```python
from build123d import *

# Parameters (mm, degrees)
SKETCH_1_R               = 2
EXTRUDE_1_DEPTH          = 15
SKETCH_2_R               = 2.5
EXTRUDE_2_DEPTH          = 4
SKETCH_3_R               = 3
EXTRUDE_3_DEPTH          = 3
SKETCH_4_R               = 9
EXTRUDE_4_DEPTH          = 3
SKETCH_5_R               = 3
EXTRUDE_5_DEPTH          = 20
SKETCH_8_R               = 2
EXTRUDE_6_DEPTH          = 4
HOLE_WIZARD_M3_2_D       = 2.5
PATTERN_CIRCULAR_2_COUNT = 4
CHAMFER_1_SIZE           = 0.3


with BuildPart() as part:
    # 草图1 → 凸台-拉伸1 (new body)
    with BuildSketch(Plane(origin=(0, 0, 0), x_dir=(0, 0, -1), z_dir=(1, 0, 0))):
        Circle(SKETCH_1_R)
    extrude(amount=EXTRUDE_1_DEPTH)

    # 草图2 → 凸台-拉伸2 (add)
    with BuildSketch(Plane(origin=(15, 0, 0), x_dir=(0, 0, -1), z_dir=(1, 0, 0))):
        Circle(SKETCH_2_R)
    extrude(amount=EXTRUDE_2_DEPTH)

    # 草图3 → 凸台-拉伸3 (add)
    with BuildSketch(Plane(origin=(19, 0, 0), x_dir=(0, 0, -1), z_dir=(1, 0, 0))):
        Circle(SKETCH_3_R)
    extrude(amount=EXTRUDE_3_DEPTH)

    # 草图4 → 凸台-拉伸4 (add)
    with BuildSketch(Plane(origin=(22, 0, 0), x_dir=(0, 0, -1), z_dir=(1, 0, 0))):
        Circle(SKETCH_4_R)
    extrude(amount=EXTRUDE_4_DEPTH)

    # 草图5 → 凸台-拉伸5 (add)
    with BuildSketch(Plane(origin=(25, 0, 0), x_dir=(0, 0, -1), z_dir=(1, 0, 0))):
        Circle(SKETCH_5_R)
    extrude(amount=EXTRUDE_5_DEPTH)

    # 草图8 → 凸台-拉伸6 (add)
    with BuildSketch(Plane(origin=(45, 0, 0), x_dir=(0, 0, -1), z_dir=(1, 0, 0))):
        Circle(SKETCH_8_R)
    extrude(amount=EXTRUDE_6_DEPTH)

    # M3 螺纹孔2 (through all)
    with Locations(Plane.ZY.offset(-22)):
        with Locations((0, 7)):
            hole_wizard_m3_2 = Hole(HOLE_WIZARD_M3_2_D / 2)

    # 阵列(圆周)2: M3 螺纹孔2 ×4 about axis
    pattern_circular_2_axis = Axis((0, 0, 0), (1, 0, 0))
    for i in range(1, PATTERN_CIRCULAR_2_COUNT):
        add(hole_wizard_m3_2.rotate(pattern_circular_2_axis, i * 360 / PATTERN_CIRCULAR_2_COUNT), mode=Mode.SUBTRACT)

    # 倒角1
    chamfer_1_edges = [part.edges().sort_by_distance(p)[0] for p in [
        (22, 0, 9),
        (0, 0, 2),
        (49, 0, 2),
    ]]
    chamfer(chamfer_1_edges, length=CHAMFER_1_SIZE)


solid = part.part
```
Check sheet for the modelled part. Datum: model origin and axes. Units: mm. A direction names the side the tool comes from. Give positions to 0.01 mm unless a question says otherwise; leave off trailing zeros. Loops run counter-clockwise (first coordinate to the right, second up) from the corner with the lowest first, then second, coordinate; pieces in that order, holes last. Notation, with made-up numbers: (57.25, 25) - (107.25, 25) arc R20 cw to (107.25, 33) - close; hole circle Ø8 at (54, 71.5). An arc over 180 degrees is marked (long way). One line per question, with ' | ' between items. Start each with the question number.
1. Draft check along Y on faces 1 (the flat face through (0, 0, 0)), 2 (the cylindrical face through (23.52, 5.78, 0.27)), 3 (the cylindrical face through (20, 0, 3)). Enter one of: released by +Y, released by -Y, zero draft, split by the parting line, or undercut.
2. Material ranges on line 1 along Y through (x, z) = (24.1, 0); line 2 along X through (y, z) = (-2.75, 7.5); line 3 along X through (y, z) = (1, -2.5), recorded low to high. Write a range as [from, to].
3. Set-up check for faces 4 (the flat face through (25, -4, 0)), 5 (the flat face through (19, 2, 2)), 6 (the cylindrical face through (23.52, -5.78, -0.27)): record each of +Z, -Z, +X, -X, +Y, -Y from which the full face is reachable in a straight line by a thin tool's end or side.
4. Cross-section at D-D, the plane x = 15.5. Enter the section's corners in (y, z).
5. Gauge pin test, flat ends, axial feed: pin 1 Ø4 at (x, z) = (17, -4) entering from -Y; pin 2 Ø3 at (y, z) = (0, 7) entering from +X; pin 3 Ø6 at (x, y) = (8, -2) entering from +Z. Record the tip position at first contact, or that the pin passes through.
6. Cross-section at C-C, the plane x = 37. Enter the section's corners in (y, z).
7. Cross-section at A-A, the plane z = 0. Give the number of separate pieces and of enclosed holes in the cut face, plus the area to 3 significant figures.
Check result:
1) face 1: zero draft | face 2: undercut | face 3: split by the parting line
2) line 1: y = [-9, -8.25], [-5.75, 5.75], [8.25, 9] | line 2: x = [22, 25] | line 3: x = [19, 45]
3) face 4: +X | face 5: -X | face 6: +X, -X
4) outline: circle Ø5 at (0, 0)
5) pin 1: stops at y = -1.5 | pin 2: stops at x = 25 | pin 3: stops at z = 2
6) outline: circle Ø6 at (0, 0)
7) separate pieces: 3 | enclosed holes: 0 | area: 273 mm2
